Build history of the part. All positions in model axes, mm. A direction names the side the tool comes from. Round coordinates to 2 decimals unless told otherwise and drop trailing zeros. Write each loop counter-clockwise with the first axis right and the second up, starting at its lowest first coordinate (ties: lowest second). Pieces come first, ordered by that corner, then holes. Notation, with made-up numbers: (-28, -3.5) - (17, -3.5) arc R24 cw to (17, 22.5) - close; hole circle Ø9 at (-29.75, -3.5). An arc over 180 degrees is marked (long way). Write each question's results on one line, items separated by ' | '.
from build123d import *

# Parameters (mm, degrees)
F0_W     = 17.78
F0_H     = 7.62
F0_R     = 2.54
F0_R_2   = 1.27
F1_DEPTH = 3.81
F2_DEPTH = 50.8
F3_DEPTH = 25.4
F4_W     = 0.363861
F4_H     = 0.363861
F5_DEPTH = 5.08
F6_W     = 0.377071
F6_H     = 0.377071
F7_DEPTH = 5.08


with BuildPart() as f1:
    # F0 (on Front) → F1 (new body)
    with BuildSketch(Plane.XZ):
        with Locations((-35.528351, 23.59897)):
            Rectangle(F0_W, F0_H)
        with Locations((-39.973351, 23.59897)):
            Circle(F0_R, mode=Mode.SUBTRACT)
        with Locations((-31.083351, 23.59897)):
            Circle(F0_R, mode=Mode.SUBTRACT)
        with Locations((-39.973351, 23.59897)):
            Circle(F0_R)
        with Locations((-39.973351, 23.59897)):
            Circle(F0_R_2, mode=Mode.SUBTRACT)
        with Locations((-39.973351, 23.59897)):
            Circle(F0_R_2)
        with Locations((-31.083351, 23.59897)):
            Circle(F0_R)
        with Locations((-31.083351, 23.59897)):
            Circle(F0_R_2, mode=Mode.SUBTRACT)
        with Locations((-31.083351, 23.59897)):
            Circle(F0_R_2)
    extrude(amount=-F1_DEPTH)

    # F0 (on Front) → F2 (join)
    with BuildSketch(Plane.XZ):
        with Locations((-39.973351, 23.59897)):
            Circle(F0_R_2)
        with Locations((-31.083351, 23.59897)):
            Circle(F0_R_2)
    extrude(amount=F2_DEPTH)

    # F0 (on Front) → F3 (join)
    with BuildSketch(Plane.XZ):
        with Locations((-39.973351, 23.59897)):
            Circle(F0_R)
        with Locations((-39.973351, 23.59897)):
            Circle(F0_R_2, mode=Mode.SUBTRACT)
        with Locations((-31.083351, 23.59897)):
            Circle(F0_R)
        with Locations((-31.083351, 23.59897)):
            Circle(F0_R_2, mode=Mode.SUBTRACT)
    extrude(amount=F3_DEPTH)

    # F4 (on face) → F5 (join)
    with BuildSketch(Plane.XZ.offset(50.8)):
        with Locations((-39.97335, 23.598971)):
            Rectangle(F4_W, F4_H)
    extrude(amount=F5_DEPTH)

    # F6 (on face) → F7 (join)
    with BuildSketch(Plane.XZ.offset(50.8)):
        with Locations((-31.08335, 23.598971)):
            Rectangle(F6_W, F6_H)
    extrude(amount=F7_DEPTH)


solid = f1.part
(1) Slice it at A-A, the plane z = 21.75. Write the cut outline in (x, y), and give its area (3 significant figures).
Worked answers:
outline: (-44.42, 0) - (-41.71, 0) - (-41.71, -25.4) - (-38.23, -25.4) - (-38.23, 0) - (-32.82, 0) - (-32.82, -25.4) - (-29.34, -25.4) - (-29.34, 0) - (-26.64, 0) - (-26.64, 3.81) - (-44.42, 3.81) - close | area: 245 mm2
(2) Two-plate mould, pull along X, no slides. Class faces 3 (the flat face through (-36, 2, 27.409)), 4 (the cylindrical face through (-33.62, -12.52, 23.71)), 5 (the flat face through (-26.638, 2, 24)): released by +X, released by -X, zero draft, split by the parting line, or undercut.
Worked answers:
face 3: zero draft | face 4: undercut | face 5: released by +X
(3) Slice it at B-B, the plane y = -10. Write the cut outline in (x, z).
Worked answers:
outline: circle Ø5.08 at (-39.97, 23.6); circle Ø5.08 at (-31.08, 23.6)
(4) Drill centre lines: probe 1 along X at (y, z) = (-9, 23.75); probe 2 along Y at (x, z) = (-34.25, 22); probe 3 along X at (y, z) = (-7, 23). Where is each one in solid material? Low to high. Write a range as [from, to].
Worked answers:
probe 1: x = [-42.51, -37.44], [-33.62, -28.55] | probe 2: y = [0, 3.81] | probe 3: x = [-42.44, -37.5], [-33.55, -28.61]
(5) Flat gauge pins, fed straight in: pin 1 Ø4 at (y, z) = (-22.5, 22) entering from +X; pin 2 Ø1 at (y, z) = (-21, 23.5) entering from -X; pin 3 Ø8 at (x, y) = (-34.5, -24.5) entering from +Z. Where does each tip first touch, or does it go through?
Worked answers:
pin 1: stops at x = -28.54 | pin 2: stops at x = -42.51 | pin 3: stops at z = 26.14
(6) Tool access for faces 1 (the flat face through (-44.418, 2, 24)), 2 (the cylindrical face through (-40.981, -37.922, 22.826)): list every direction of +Z, -Z, +X, -X, +Y, -Y with a clear straight run to the whole face (end or side of a thin tool).
Worked answers:
face 1: +Z, -Z, -X, +Y, -Y | face 2: -Y
(7) Slice it at C-C, the plane x = -33. Write the cut outline in (y, z), and give its area (3 significant figures).
Worked answers:
outline: (-25.4, 21.93) - (0, 21.93) - (0, 19.79) - (3.81, 19.79) - (3.81, 27.41) - (0, 27.41) - (0, 25.27) - (-25.4, 25.27) - close | area: 114 mm2
(8) Slice it at D-D, the plane z = 26.75. Write the cut outline in (x, y), and give its area (3 significant figures).
Worked answers:
outline: (-44.42, 0) - (-26.64, 0) - (-26.64, 3.81) - (-44.42, 3.81) - close | area: 67.7 mm2
